```python
from build123d import *

# Parameters (mm, degrees)
BOSS_EXTRUDE1_DEPTH = 6
SKETCH3_R           = 1.75
CUT_EXTRUDE2_DEPTH  = 67.08422656
BOSS_EXTRUDE2_DEPTH = 12
BOSS_EXTRUDE3_DEPTH = 6
CUT_EXTRUDE3_REACH  = 72.051
SKETCH6_R           = 1.75
CUT_EXTRUDE4_REACH  = 72.051
SKETCH8_R           = 12.25
BOSS_EXTRUDE4_DEPTH = 11
SKETCH9_R           = 2.55
SKETCH9_R_2         = 3
CUT_EXTRUDE5_DEPTH  = 6


with BuildPart() as part:
    # Sketch1 → Boss-Extrude1 (new body)
    with BuildSketch(Plane(origin=(0, 0, 0), x_dir=(1, 0, 0), z_dir=(0, 1, 0))):
        with BuildLine():
            Line((-50, 14.25), (50, 14.25))
            ThreePointArc((50, 14.25), (64.25, 0), (50, -14.25))
            Line((50, -14.25), (-50, -14.25))
            ThreePointArc((-50, -14.25), (-64.25, 0), (-50, 14.25))
        make_face()
    extrude(amount=BOSS_EXTRUDE1_DEPTH)

    # Sketch3 → Cut-Extrude2 (cut, through all)
    with BuildSketch(Plane.XZ):
        with Locations(Location((50, 0, 0), (0, 0, 270))):
            Circle(SKETCH3_R)
    extrude(amount=-CUT_EXTRUDE2_DEPTH, mode=Mode.SUBTRACT)

    # Sketch4 → Boss-Extrude2 (add)
    with BuildSketch(Plane(origin=(0, 6, 0), x_dir=(1, 0, 0), z_dir=(0, 1, 0))):
        with BuildLine():
            Line((-50, 14.25), (15, 14.25))
            Line((15, 14.25), (15, -14.25))
            Line((15, -14.25), (-50, -14.25))
            ThreePointArc((-50, -14.25), (-64.25, 0), (-50, 14.25))
        make_face()
    extrude(amount=BOSS_EXTRUDE2_DEPTH)

    # Sketch5 → Boss-Extrude3 (add)
    with BuildSketch(Plane(origin=(0, 18, 0), x_dir=(1, 0, 0), z_dir=(0, 1, 0))):
        with BuildLine():
            Line((-50, 14.25), (50, 14.25))
            ThreePointArc((50, 14.25), (64.25, 0), (50, -14.25))
            Line((50, -14.25), (-50, -14.25))
            ThreePointArc((-50, -14.25), (-64.25, 0), (-50, 14.25))
        make_face()
    extrude(amount=BOSS_EXTRUDE3_DEPTH)

    # Sketch6 → Cut-Extrude3 (cut, up to next)
    with BuildSketch(Plane(origin=(0, 24, 0), x_dir=(1, 0, 0), z_dir=(0, 1, 0)), mode=Mode.PRIVATE) as cut_extrude3_sk1:
        with Locations(Location((50, 0, 0), (0, 0, 90))):
            Circle(SKETCH6_R)
    cut_extrude3_tool1 = extrude(cut_extrude3_sk1.sketch, amount=-CUT_EXTRUDE3_REACH, mode=Mode.PRIVATE) & part.part
    add(cut_extrude3_tool1.solids().sort_by_distance((50, 24, 0))[0], mode=Mode.SUBTRACT)

    # Sketch7 → Cut-Extrude4 (cut, up to next)
    with BuildSketch(Plane(origin=(0, 24, 0), x_dir=(1, 0, 0), z_dir=(0, 1, 0)), mode=Mode.PRIVATE) as cut_extrude4_sk1:
        with BuildLine():
            ThreePointArc((-39.07315683, -9.146944754), (-43.970135273, -12.911360555), (-50, -14.25))
            Line((-50, -14.25), (50, -14.25))
            add(Edge.make_bspline(
                [(-39.07315683, -9.146944754), (-31.514094033, -0.116968526), (5.438655837, -4.645240543), (38.697514387, -14.25), (50, -14.25)],
                knots=[0, 0, 0, 0, 0.435907903, 1, 1, 1, 1], degree=3))
        make_face()
    cut_extrude4_tool1 = extrude(cut_extrude4_sk1.sketch, amount=-CUT_EXTRUDE4_REACH, mode=Mode.PRIVATE) & part.part
    add(cut_extrude4_tool1.solids().sort_by_distance((-8.590717, 24, 9.791359))[0], mode=Mode.SUBTRACT)

    # Sketch8 → Boss-Extrude4 (add)
    with BuildSketch(Plane.XZ):
        with Locations(Location((-50, 0, 0), (0, 0, 90))):
            Circle(SKETCH8_R)
    extrude(amount=BOSS_EXTRUDE4_DEPTH)

    # Sketch9 → Cut-Extrude5 (cut)
    with BuildSketch(Plane.XZ.offset(11)):
        with Locations(Location((-50, 6.75, 0), (0, 0, 270))):
            Circle(SKETCH9_R)
        with Locations(Location((-50, -6.75, 0), (0, 0, 270))):
            Circle(SKETCH9_R)
        with Locations(Location((-50, 0, 0), (0, 0, 270))):
            Circle(SKETCH9_R_2)
    extrude(amount=-CUT_EXTRUDE5_DEPTH, mode=Mode.SUBTRACT)


solid = part.part
```
Can you work these out from the model? Positions are in its coordinate system, mm. A direction names the side the tool comes from. Give positions to 0.01 mm unless a question says otherwise; leave off trailing zeros. Write each loop counter-clockwise with the first axis right and the second up, starting at its lowest first coordinate (ties: lowest second). Pieces come first, ordered by that corner, then holes. Notation, with made-up numbers: (12, -15) - (20, -15) arc R24 ccw to (20, -5) - close; hole circle Ø7 at (21.5, -24). An arc over 180 degrees is marked (long way). Write item = value, one per line. Start each with the question number.
1. Please list where these lines run through material, in increasing order: line 1 (X direction, y = 19.4, z = 0); line 2 (Y direction, x = 33.5, z = -8); line 3 (Y direction, x = 11, z = -5.25).
2. On a 3-axis mill with a long thin cutter (end or side, diameter ignored), from which of +Z, -Z, +X, -X, +Y, -Y can I reach the whole of each face in a straight line? I mean faces 1 (the face through (-47, -8, 0)), 2 (the face through (40, 18, 0)), 3 (the face through (1, 24, -3)). Say none if no direction works.
3. Imagine slicing it at A-A (z = 0). Please give me the cut outline in (x, y), and give its area (3 significant figures).
4. Imagine slicing it at B-B (y = -3.5). Please give me the cut outline in (x, z).
5. For pin 1 (6 mm diameter, centred on y = 9.5, z = 9, fed in from +X); pin 2 (1.5 mm diameter, centred on x = -50, z = -7.5, fed in from -Y); pin 3 (2 mm diameter, centred on x = 50, z = 0, fed in from +Y); pin 4 (6 mm diameter, centred on y = 11, z = -5.5, fed in from -X), each with a flat end and sliding along its axis, tell me the tip position at first contact or that it passes through.
6. Thinking about a two-plate mould opening in Z: for faces 4 (the face through (15, 0, -3)), 5 (the face through (-47.85, -8.04, -8.12)), 6 (the face through (64.247, 2.958, -0.313)), which applies, released by +Z, released by -Z, zero draft, split by the parting line, or undercut?
Worked answers:
q1.line_1 = -64.25 to 48.25, 51.75 to 64.25
q1.line_2 = 0 to 6, 18 to 24
q1.line_3 = 0 to 24
q2.face_1 = -Y
q2.face_2 = +Z, -Z, +X
q2.face_3 = +Z, -Z, +X, -X, +Y
q3.outline = (-64.25, 0) - (-62.25, 0) - (-62.25, -11) - (-53, -11) - (-53, -5) - (-47, -5) - (-47, -11) - (-37.75, -11) - (-37.75, 0) - (48.25, 0) - (48.25, 6) - (15, 6) - (15, 18) - (48.25, 18) - (48.25, 24) - (-64.25, 24) - close; (51.75, 0) - (64.25, 0) - (64.25, 6) - (51.75, 6) - close; (51.75, 18) - (64.25, 18) - (64.25, 24) - (51.75, 24) - close
q3.area = 2,680 mm2
q4.outline = circle Ø24.5 at (-50, 0)
q5.pin_1 = 15
q5.pin_2 = -5
q5.pin_3 = through
q5.pin_4 = -64.03
q6.face_4 = zero draft
q6.face_5 = undercut
q6.face_6 = split by the parting line
